The figure shows three views and two pictorial views of one solid part (mm, origin at its lowest corner). Answer the questions. A direction names the side the tool comes from. Round coordinates to 2 decimals unless told otherwise and drop trailing zeros. Write each loop counter-clockwise with the first axis right and the second up, starting at its lowest first coordinate (ties: lowest second). Pieces come first, ordered by that corner, then holes. Notation, with made-up numbers: M 39.25,54.25 L 64.25,54.25 A19 cw 64.25,77.25 Z; hole C 7,55.25 d1. An arc over 180 degrees is marked long. One line per item, written item: value. Start each with the question number.
Q1. Given pin 1 Ø1.5 at (y, z) = (4, 3.5) entering from +X, flat-ended and moving along its own axis, determine where the tip first touches the part or whether it passes through.
Q2. Find section D-D (z = 0.75). Write down the section's boundary in (x, y).
Q3. Find section B-B (z = 3.5). Write down the section's boundary in (x, y) (3 decimals).
Q4. Consider probe 1 along Y at (x, z) = (18, 3.5) (3 decimals); probe 2 along Z at (x, y) = (15, 6.5); probe 3 along Y at (x, z) = (17, 2.5). Determine where each line is inside the solid, lowest interval first.
Q5. A tool of negligible diameter and unlimited length cuts with its end or side. For the marked faces 1 and 2, from which of +Z, -Z, +X, -X, +Y, -Y can it reach the whole face along a straight path? Write none if from no direction.
Q6. Find section A-A (y = 6.6). Write down the section's boundary in (x, z) (3 decimals).
Q7. Find section C-C (x = 26). Write down the section's boundary in (y, z), and give its area (3 significant figures).
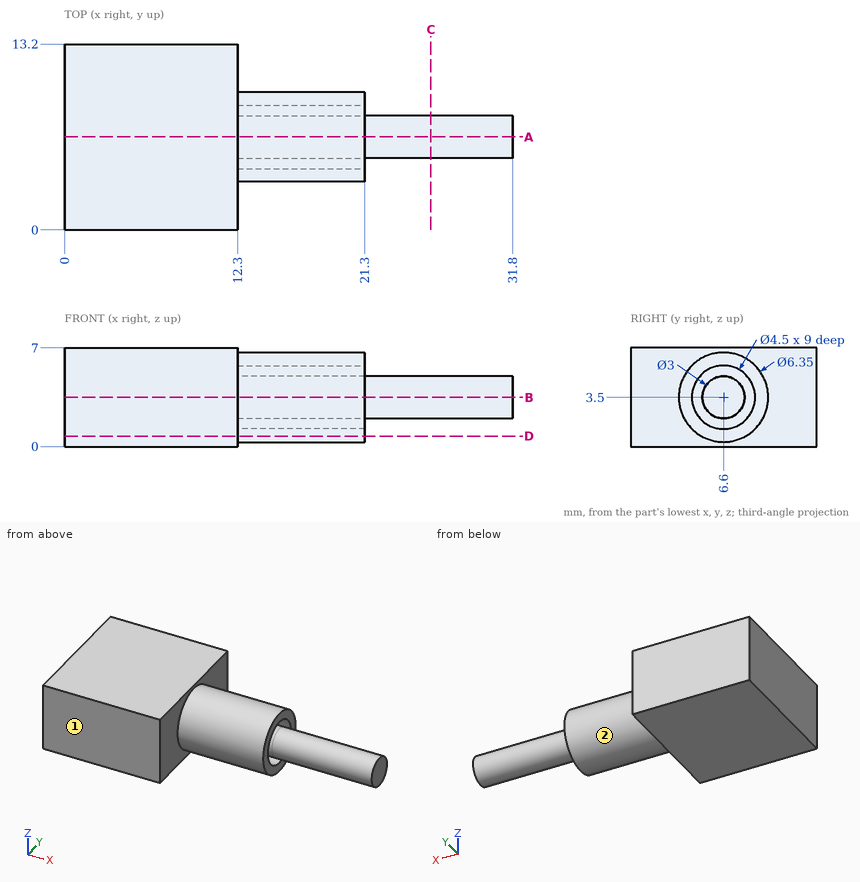
The answers:
1. pin 1: x = 21.3
2. outline: M 0,0 L 12.3,0 L 12.3,5.01 L 21.3,5.01 L 21.3,8.19 L 12.3,8.19 L 12.3,13.2 L 0,13.2 Z
3. outline: M 0,0 L 12.3,0 L 12.3,3.425 L 21.3,3.425 L 21.3,4.35 L 12.3,4.35 L 12.3,5.1 L 31.8,5.1 L 31.8,8.1 L 12.3,8.1 L 12.3,8.85 L 21.3,8.85 L 21.3,9.775 L 12.3,9.775 L 12.3,13.2 L 0,13.2 Z
4. probe 1: 3.425 to 4.35, 5.1 to 8.1, 8.85 to 9.775
4. probe 2: 0.33 to 1.25, 2 to 5, 5.75 to 6.67
4. probe 3: 3.59 to 4.58, 5.48 to 7.72, 8.62 to 9.61
5. face 1: +Z, -Z, +X, -X, -Y
5. face 2: +X
6. outline: M 0,0 L 12.3,0 L 12.3,0.325 L 21.3,0.325 L 21.3,1.25 L 12.3,1.25 L 12.3,2 L 31.8,2 L 31.8,5 L 12.3,5 L 12.3,5.75 L 21.3,5.75 L 21.3,6.675 L 12.3,6.675 L 12.3,7 L 0,7 Z
7. outline: C 6.6,3.5 d3
7. area: 7.07 mm2
